Could you check a few things on this drawing? It's one solid part, dimensions in mm from its lowest x, y, z. A direction names the side the tool comes from. Round coordinates to 2 decimals unless told otherwise and drop trailing zeros. Loops run counter-clockwise (first coordinate to the right, second up) from the corner with the lowest first, then second, coordinate; pieces in that order, holes last. Notation, with made-up numbers: (76.25, 27) -> (113.25, 27) arc R24 cw to (113.25, 56) -> close; hole circle Ø1 at (88.25, 66). An arc over 180 degrees is marked (long way). Use CSV: the item, a comma, the result in double quotes. Start each with the question number.
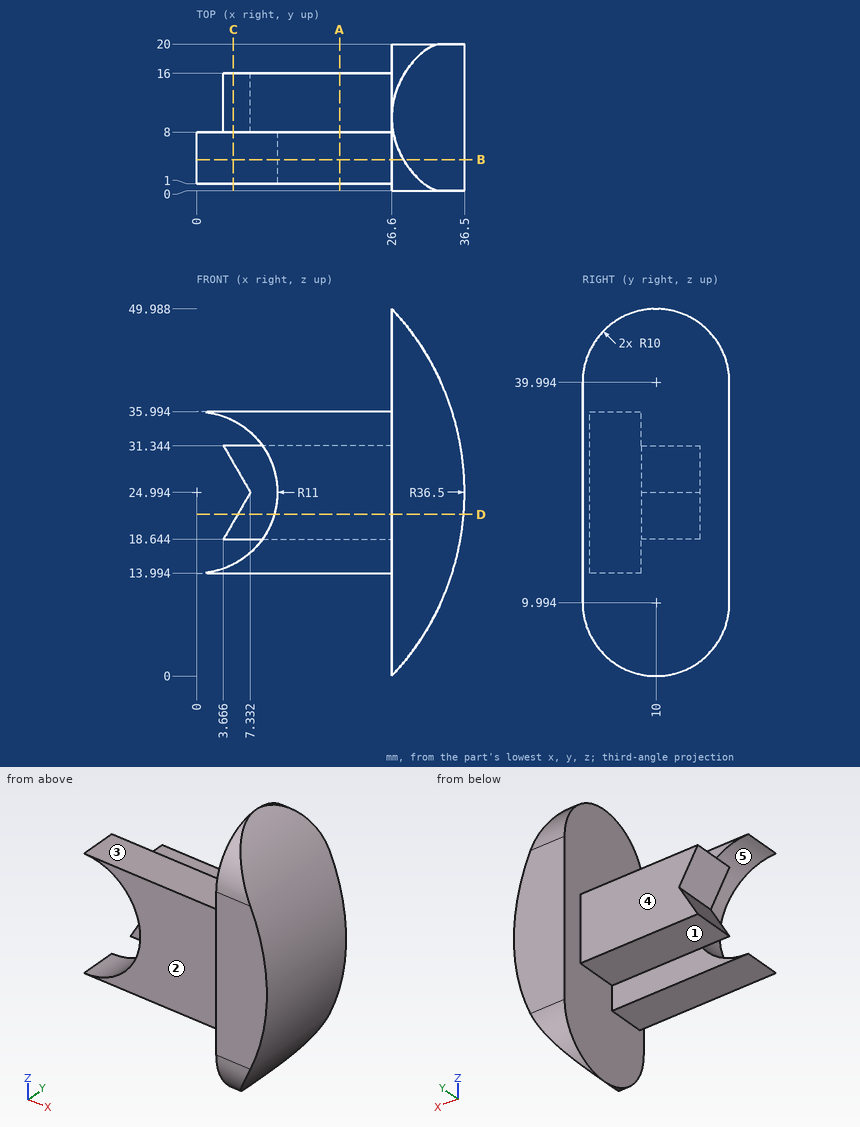
Q1. For the marked faces 1, 2, 3, 4 and 5, which set-ups out of +Z, -Z, +X, -X, +Y, -Y let a thin tool reach every point of the face, with its end or its side?
Q2. I want a section at C-C, the plane x = 5. List the corners of the cut face in (y, z) for me.
Q3. I want a section at D-D, the plane z = 22. List the corners of the cut face in (x, y) for me (1 decimal), then the cut area to 3 significant figures.
Q4. I want a section at B-B, the plane y = 4.25. List the corners of the cut face in (x, z) for me (1 decimal), then the cut area to 3 significant figures.
Q5. I need wall thicknesses on line 1 along Z through (x, y) = (21, 9.75); line 2 along Z through (x, y) = (3.5, 4.75) (1 decimal); line 3 along Z through (x, y) = (18, 5). Which ranges of each line are inside material? Lowest first, please.
Q6. I want a section at A-A, the plane x = 19.5. List the corners of the cut face in (y, z) for me, then the cut area to 3 significant figures.
Q7. Will these pins go through, and if not, where does the flat tip stop? pin 1 Ø5 at (x, z) = (12, 16) entering from +Y; pin 2 Ø10 at (x, z) = (20, 22) entering from +Y; pin 3 Ø10 at (x, y) = (29, 11) entering from -Z; pin 4 Ø1.5 at (y, z) = (14.5, 12.5) entering from +X.
Values found:
1,face 1,"-Z, -X, +Y"
1,face 2,"+Z, -Z, -X, -Y"
1,face 3,"+Z, -X, +Y, -Y"
1,face 4,"+Z, -Z, -X, +Y"
1,face 5,"-X, -Y"
2,outline,"(1, 13.99) -> (8, 13.99) -> (8, 15.2) -> (1, 15.2) -> close; (1, 34.79) -> (8, 34.79) -> (8, 35.99) -> (1, 35.99) -> close; (8, 18.64) -> (16, 18.64) -> (16, 20.95) -> (8, 20.95) -> close; (8, 29.03) -> (16, 29.03) -> (16, 31.34) -> (8, 31.34) -> close"
3,outline,"(5.6, 8) -> (10.6, 8) -> (10.6, 1) -> (26.6, 1) -> (26.6, 0) -> (36.4, 0) -> (36.4, 20) -> (26.6, 20) -> (26.6, 16) -> (5.6, 16) -> close"
3,area,"476 mm2"
4,outline,"(0, 14) -> (26.6, 14) -> (26.6, 1.8) -> (28.2, 1.8) arc R36.5 ccw to (28.2, 48.2) -> (26.6, 48.2) -> (26.6, 36) -> (0, 36) arc R11 cw to start"
4,area,"732 mm2"
5,line 1,"18.64 to 31.34"
5,line 2,"14 to 14.6, 35.4 to 36"
5,line 3,"13.99 to 35.99"
6,outline,"(1, 13.99) -> (8, 13.99) -> (8, 18.64) -> (16, 18.64) -> (16, 31.34) -> (8, 31.34) -> (8, 35.99) -> (1, 35.99) -> close"
6,area,"256 mm2"
7,pin 1,"y = 8"
7,pin 2,"y = 16"
7,pin 3,"z = 0"
7,pin 4,"x = 34.56"
